Autodesk Fusion 360 part; units mm, degrees
sketch "Sketch1" plane through (0, 0, 0) normal (0, 0, 1) x (1, 0, 0)
  circle A0 centre (0, 0) radius 2.95
  dimension "d1" = 5.9
extrude "Extrude1" add sketch "Sketch1" along normal blind 12
sketch "Sketch2" plane through (0, 0, 12) normal (0, 0, 1) x (-1, 0, 0)
  circle A0 centre (0, 0) radius 2.95
  circle A1 centre (0, 0) radius 4.084
extrude "Extrude2" add sketch "Sketch2" along normal blind 3 contours A0 | A1
sketch "Sketch3" plane through (0, 0, 15) normal (0, 0, 1) x (-1, 0, 0)
  circle A0 centre (0, 0) radius 4.084
  circle A1 centre (0, 0) radius 1.75
  dimension "d6" = 3.5
extrude "Extrude3" cut sketch "Sketch3" against normal blind 4 contours A1
Read the model definition and answer for the solid it produces. Units are mm, in the model's axes. A direction names the side the tool comes from. Round coordinates to 2 decimals unless told otherwise and drop trailing zeros. Loops run counter-clockwise (first coordinate to the right, second up) from the corner with the lowest first, then second, coordinate; pieces in that order, holes last.
Q1. Section D-D on z = 1.75 is taken. Write down the section's boundary in (x, y).
Q2. Determine the mould class of faces 3 (the face through (0, 0, 11)), 4 (the face through (-1, 3, 12)), 5 (the face through (-2.947, -0.13, 5.916)) for opening direction Y: released by +Y, released by -Y, zero draft, split by the parting line, or undercut.
Q3. Section A-A on z = 11.75 is taken. Write down the section's boundary in (x, y), and give its area (3 significant figures).
Q4. Section B-B on y = 0 is taken. Write down the section's boundary in (x, z), and give its area (3 significant figures).
Q5. Each of these flat-tipped pins is pushed along its axis until it touches: pin 1 (1.5 mm diameter, centred on x = 1.5, z = 7, fed in from -Y); pin 2 (1.5 mm diameter, centred on x = 2, z = 5, fed in from +Y); pin 3 (3 mm diameter, centred on x = 0, y = 0, fed in from +Z); pin 4 (3 mm diameter, centred on x = 0, y = -0.5, fed in from +Z). Where does it stop, or does it pass through?
Q6. Consider probe 1 along X at (y, z) = (0, 12.35); probe 2 along Z at (x, y) = (3, 2.25). Determine where each line is inside the solid, lowest interval first.
Q7. Which of the six approach directions +Z, -Z, +X, -X, +Y, -Y give full straight-line access (tool end or side, diameter ignored) to faces 1 (the face through (-1.617, 0.67, 13.028)), 2 (the face through (0, 0, 0))?
Output:
1. outline: circle Ø5.9 at (0, 0)
2. face 3: undercut
2. face 4: zero draft
2. face 5: split by the parting line
3. outline: circle Ø5.9 at (0, 0); hole circle Ø3.5 at (0, 0)
3. area: 17.7 mm2
4. outline: (-4.08, 12) - (-2.95, 12) - (-2.95, 0) - (2.95, 0) - (2.95, 12) - (4.08, 12) - (4.08, 15) - (1.75, 15) - (1.75, 11) - (-1.75, 11) - (-1.75, 15) - (-4.08, 15) - close
4. area: 81.3 mm2
5. pin 1: stops at y = -2.85
5. pin 2: stops at y = 2.67
5. pin 3: stops at z = 11
5. pin 4: stops at z = 15
6. probe 1: x = -4.08 to -1.75, 1.75 to 4.08
6. probe 2: z = 12 to 15
7. face 1: +Z
7. face 2: -Z, +X, -X, +Y, -Y
